Autodesk Inventor part; units mm, degrees
ref_plane "YZ Plane" through (0, 0, 0) normal (1, 0, 0) x (0, 1, 0)
ref_plane "XZ Plane" through (0, 0, 0) normal (0, 1, 0) x (-1, 0, 0)
ref_plane "XY Plane" through (0, 0, 0) normal (0, 0, 1) x (1, 0, 0)
sketch "Sketch1" plane through (0, 0, 0) normal (0, 0, 1) x (1, 0, 0)
  line L0 (12.7, 25.4) -> (-12.7, 25.4)
  line L1 (-12.7, 25.4) -> (-12.7, -25.4)
  line L2 (-12.7, -25.4) -> (12.7, -25.4)
  line L3 (12.7, -25.4) -> (12.7, 25.4)
  line L4 (12.7, 25.4) -> (-12.7, -25.4) construction
  line L5 (-12.7, 25.4) -> (12.7, -25.4) construction
  line L6 (-11.684, 24.384) -> (11.684, 24.384)
  line L7 (11.684, 24.384) -> (11.684, -24.384)
  line L8 (11.684, -24.384) -> (-11.684, -24.384)
  line L9 (-11.684, -24.384) -> (-11.684, 24.384)
  point P0 (0, 0)
  dimension "d0" = 1.016
  dimension "d1" = 50.8
  dimension "d2" = 25.4
extrude "Tube Length" add sketch "Sketch1" along normal mid plane 190.5
sketch "Sketch2" plane through (-12.7, 25.4, 95.25) normal (0, 1, 0) x (1, 0, 0)
  line L0 (0, 0) -> (0, 190.5)
  line L1 (25.4, 0) -> (0, 0)
  line L2 (25.4, 190.5) -> (25.4, 0)
  line L3 (0, 190.5) -> (25.4, 190.5)
  line L4 (25.4, 0) -> (0, 0)
  line L5 (12.7, 0) -> (12.7, 12.7) construction
  circle A0 centre (12.7, 12.7) radius 2.2479
  point P0 (12.7, 95.25)
  dimension "d5" = 12.7
  dimension "d6" = 4.4958
extrude "Top Hole" cut sketch "Sketch2" against normal through all contours A0
pattern_linear "Rectangular Pattern1" count 8 spacing 25.4 along (0, 0, -1) of "Top Hole"
sketch "Sketch3" plane through (0, 0, 95.25) normal (0, 0, 1) x (1, 0, 0)
  line L0 (0, 0) -> (0, 25.4) construction
  line L1 (12.7, 25.4) -> (-12.7, 25.4)
  line L2 (-0.0508, 25.4) -> (0, 25.2984)
  line L3 (0.0508, 25.4) -> (0, 25.2984)
  line L4 (-12.7, 12.6492) -> (-12.5984, 12.7)
  line L5 (-12.7, 12.7508) -> (-12.5984, 12.7)
  line L6 (-12.7, -0.0508) -> (-12.5984, 0)
  line L7 (-12.7, 0.0508) -> (-12.5984, 0)
  line L8 (-12.7, -12.7508) -> (-12.5984, -12.7)
  line L9 (-12.7, -12.6492) -> (-12.5984, -12.7)
  line L10 (12.7, 0.0508) -> (12.5984, 0)
  line L11 (12.7, 12.6492) -> (12.5984, 12.7)
  line L12 (12.7, 12.7508) -> (12.5984, 12.7)
  line L13 (12.7, -0.0508) -> (12.5984, 0)
  line L14 (12.7, -12.6492) -> (12.5984, -12.7)
  line L15 (12.7, -12.7508) -> (12.5984, -12.7)
  line L16 (0.0508, -25.4) -> (0, -25.2984)
  line L17 (-0.0508, -25.4) -> (0, -25.2984)
  line L18 (-12.7, 25.4) -> (-12.7, -25.4)
  line L19 (12.7, -25.4) -> (12.7, 25.4)
  line L20 (-12.7, -25.4) -> (12.7, -25.4)
  point P0 (0, 12.7)
  point P1 (-12.7, 12.7)
  point P2 (-12.7, 0)
  point P3 (-12.7, -12.7)
  point P4 (12.7, 12.7)
  point P5 (12.7, 0)
  point P6 (12.7, -12.7)
  point P7 (0, -25.4)
  dimension "d12" = 0.1016
  dimension "d13" = 0.1016
  dimension "d16" = 90
  dimension "d20" = 12.7
  dimension "d27" = 360
equation "\"d13\" = d12"
properties part number "Stage 2 Bottom & Top Tube" material "Aluminum 6061"
Model file for the job. Use its own axes, mm. A direction names the side the tool comes from. Give positions to 0.01 mm unless a question says otherwise; leave off trailing zeros. Order: outer loops, then holes, each group sorted by start corner. A loop starts at its lowest first (then second) coordinate and runs counter-clockwise, first axis right, second up. Notation, with made-up numbers: (27, 26.5) - (51, 26.5) arc R20 cw to (51, 61.5) - close; hole circle Ø10 at (39, 14.25). An arc over 180 degrees is marked (long way). Write item = value, one per line. Start each with the question number.
1. Two-plate mould, pull along Y, no slides. Class faces 1 (the flat face through (0, -25.4, -1)), 2 (the flat face through (11.684, 0, -1)), 3 (the cylindrical face through (1.208, 24.899, -46.345)): pulls with the +Y half, pulls with the -Y half, needs draft (parallel to the pull), parting line crosses it, or undercut.
2. Drop flat-ended pins along their axis: P1, Ø7, axis at x = 0, z = 6.35, coming from the +Y side; P2, Ø3.5, axis at x = 0, z = -69.85, coming from the +Y side. Give the stop position or say it passes through.
3. Which spindle directions (+Z, -Z, +X, -X, +Y, -Y) get a long thin tool onto all of the face, cutting with end or side? Do faces 4 (the cylindrical face through (-1.78, -24.88, 7.72)), 5 (the flat face through (0, 24.384, -1)). Say none if no direction does.
4. Cut at C-C, the plane z = 23. List the corners of the cut face in (x, y).
5. Cut at A-A, the plane y = -4.5. List the corners of the cut face in (x, z).
6. Probe line 1 along X through (y, z) = (24, -19); line 2 along Y through (x, z) = (-3, 6); line 3 along X through (y, z) = (24.9, -69.85). List the from-to ranges inside material, lowest first.
7. Cut at B-B, the plane x = 10. List the corners of the cut face in (y, z), and give its area (3 significant figures).
8. Cut at D-D, the plane z = -19.05. List the corners of the cut face in (x, y), and give its area (3 significant figures).
Taken from the geometry:
q1.face_1 = pulls with the -Y half
q1.face_2 = undercut
q1.face_3 = needs draft
q2.P1 = 25.4
q2.P2 = through
q3.face_4 = +Y, -Y
q3.face_5 = +Z, -Z
q4.outline = (-12.7, -25.4) - (12.7, -25.4) - (12.7, 25.4) - (-12.7, 25.4) - close; hole (-11.68, -24.38) - (11.68, -24.38) - (11.68, 24.38) - (-11.68, 24.38) - close
q5.outline = (-12.7, -95.25) - (-11.68, -95.25) - (-11.68, 95.25) - (-12.7, 95.25) - close; (11.68, -95.25) - (12.7, -95.25) - (12.7, 95.25) - (11.68, 95.25) - close
q6.line_1 = -12.7 to -11.68, 11.68 to 12.7
q6.line_2 = -25.4 to -24.38, 24.38 to 25.4
q6.line_3 = -12.7 to -2.25, 2.25 to 12.7
q7.outline = (-25.4, -95.25) - (-24.38, -95.25) - (-24.38, 95.25) - (-25.4, 95.25) - close; (24.38, -95.25) - (25.4, -95.25) - (25.4, 95.25) - (24.38, 95.25) - close
q7.area = 387 mm²
q8.outline = (-12.7, -25.4) - (-2.25, -25.4) - (-2.25, -24.38) - (-11.68, -24.38) - (-11.68, 24.38) - (-2.25, 24.38) - (-2.25, 25.4) - (-12.7, 25.4) - close; (2.25, -25.4) - (12.7, -25.4) - (12.7, 25.4) - (2.25, 25.4) - (2.25, 24.38) - (11.68, 24.38) - (11.68, -24.38) - (2.25, -24.38) - close
q8.area = 142 mm²
